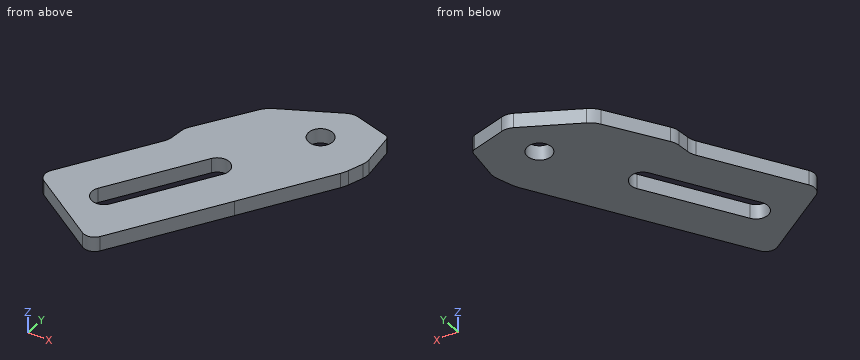
Autodesk Inventor part; units mm, degrees
ref_plane "YZ Plane" through (0, 0, 0) normal (1, 0, 0) x (0, 1, 0)
ref_plane "XZ Plane" through (0, 0, 0) normal (0, 1, 0) x (-1, 0, 0)
ref_plane "XY Plane" through (0, 0, 0) normal (0, 0, 1) x (1, 0, 0)
sketch "Body" plane through (0, 0, 0) normal (0, 0, 1) x (1, 0, 0)
  line L0 (27.316, 36.0942) -> (2.7256, -1.7701) construction
  line L1 (-2.7256, 1.7701) -> (21.8647, 39.6345) construction
  line L2 (39.19, 35.3599) -> (32.4946, 58.4071) construction
  line L3 (32.4946, 58.4071) -> (19.5232, 59.2689) construction
  line L4 (19.5232, 59.2689) -> (15.4488, 53.2513) construction
  arc A0 (15.4488, 53.2513) -> (14.6202, 51.0054) centre (19.5891, 50.448) ccw
  line L5 (14.6202, 51.0054) -> (14.2763, 47.9393)
  arc A1 (13.5008, 45.7735) -> (14.2763, 47.9393) centre (9.3074, 48.4968) ccw
  line L6 (13.5008, 45.7735) -> (-11.4127, 7.4118) construction
  line L7 (11.4127, -7.4118) -> (39.19, 35.3599) construction
  line L8 (-11.4127, 7.4118) -> (11.4127, -7.4118) construction
  arc A2 (53.351, 57.1651) -> (54.2815, 59.0478) centre (45.8031, 62.067) ccw
  arc A3 (27.3464, 69.3874) -> (24.9347, 67.2614) centre (30.251, 63.6618) ccw
  arc A4 (45.1456, 77.1234) -> (42.0612, 76.8523) centre (43.9732, 72.7788) ccw
  arc A5 (54.9347, 73.4976) -> (53.8348, 74.7787) centre (53.444, 73.3305) ccw
  arc A6 (55.6234, 62.816) -> (55.882, 65.0506) centre (50.9132, 64.4933) ccw
  line L9 (42.0612, 76.8523) -> (27.3464, 69.3874)
  line L10 (53.8348, 74.7787) -> (45.1456, 77.1234)
  line L11 (55.882, 65.0506) -> (54.9347, 73.4976)
  line L12 (54.2815, 59.0478) -> (55.6234, 62.816)
  line L13 (39.19, 35.3599) -> (53.351, 57.1651)
  arc A7 (15.4488, 53.2513) -> (14.6202, 51.0054) centre (19.5891, 50.448) ccw
  line L14 (14.6202, 51.0054) -> (14.2763, 47.9393)
  line L15 (13.5008, 45.7735) -> (-3.2428, 19.9917)
  line L16 (-3.2428, 19.9917) -> (19.5825, 5.1682)
  line L17 (19.5825, 5.1682) -> (39.19, 35.3599)
  line L18 (24.9347, 67.2614) -> (15.4488, 53.2513)
  line L19 (27.316, 36.0942) -> (21.8647, 39.6345) construction
  circle A8 centre (13.6164, 20.9665) radius 3.25
  line L20 (13.6164, 20.9665) -> (34.175, 52.6228) construction
  circle A9 centre (28.7285, 44.2362) radius 3.25
  line L21 (26.0028, 46.0064) -> (10.8907, 22.7366)
  line L22 (31.4541, 42.4661) -> (16.342, 19.1964)
  circle A10 centre (42.1456, 66.1234) radius 3.25
  point P0 (0, 0)
  point P1 (0, 0)
  dimension "d25" = 138
  dimension "d26" = 111.5
  dimension "d27" = 154
  dimension "d31" = 6.5
  dimension "d32" = 15
  dimension "d33" = 16.5
  dimension "d34" = 151
  dimension "d35" = 6.4202
  dimension "d36" = 8.5
  dimension "d37" = 4
  dimension "d38" = 9
  dimension "d39" = 4.5
  dimension "d40" = 1.5
  dimension "d41" = 5
  dimension "d42" = 9
  dimension "d43" = 26
  dimension "d44" = 6.5
  dimension "d45" = 10
  dimension "d46" = 10
  dimension "d47" = 6.5
  dimension "d48" = 3
  dimension "d49" = 11
extrude "BodyFeature" add sketch "Body" along normal blind 4
fillet "EndFilletsFeature" radius 3 2 edges at (-3.2428, 19.9917, 2) (19.5825, 5.1682, 2)
properties part number "PelvisSubLinkLeft"
Could you check a few things on this model? Use its own coordinates, in mm. Round coordinates to 2 decimals unless told otherwise and drop trailing zeros. Order: outer loops, then holes, each group sorted by start corner. A loop starts at its lowest first (then second) coordinate and runs counter-clockwise, first axis right, second up.
(1) Imagine slicing it at C-C (y = 16). Write out the boundary of the cut face in (x, z), plus the area to 3 significant figures.
Response values:
outline: (2.9, 0) - (26.62, 0) - (26.62, 4) - (2.9, 4) - close
area: 94.9 mm2
(2) Imagine slicing it at A-A (x = 19). Write out the boundary of the cut face in (y, z).
Response values:
outline: (6.33, 0) - (23.29, 0) - (23.29, 4) - (6.33, 4) - close; (35.22, 0) - (58.5, 0) - (58.5, 4) - (35.22, 4) - close
(3) Imagine slicing it at B-B (y = 40). Write out the boundary of the cut face in (x, z), plus the area to 3 significant figures.
Response values:
outline: (9.75, 0) - (22.1, 0) - (22.1, 4) - (9.75, 4) - close; (29.85, 0) - (42.2, 0) - (42.2, 4) - (29.85, 4) - close
area: 98.8 mm2
(4) Please list where these lines run through material, in increasing order: line 1 along Y through (x, z) = (42, 2.25); line 2 along X through (y, z) = (43.5, 1.55); line 3 along X through (y, z) = (22.5, 2.9).
Response values:
line 1: y = 39.69 to 62.88, 69.37 to 76.82
line 2: x = 12.02 to 24.38, 31.89 to 44.48
line 3: x = -1.61 to 10.75, 18.49 to 30.84
(5) I'm going to push flat-ended pins straight in: pin 1 (5 mm diameter, centred on x = 42.15, y = 66.12, fed in from -Z); pin 2 (1.5 mm diameter, centred on x = 23, z = 1, fed in from +Y). Where does each tip first touch, or does it pass through?
Response values:
pin 1: passes through
pin 2: stops at y = 65.51
(6) Imagine slicing it at D-D (x = 4.5). Write out the boundary of the cut face in (y, z), plus the area to 3 significant figures.
Response values:
outline: (14.96, 0) - (31.91, 0) - (31.91, 4) - (14.96, 4) - close
area: 67.8 mm2
